Geometry: see drawing. Coordinates: mm, zero at the bounding-box minimum. Coordinates: 2 decimals unless noted, no trailing zeros. Write each loop counter-clockwise with the first axis right and the second up, starting at its lowest first coordinate (ties: lowest second). Pieces come first, ordered by that corner, then holes. Notation, with made-up numbers: M 55,-32.75 L 67,-32.75 A21 ccw 67,-14.75 Z; hole C 67,-24 d11. An arc over 180 degrees is marked long. Answer as CSV lines item,"result". Start each with the question number.
1. Section B-B on z = 3.5. Return the cut outline in (x, y).
2. Mould query, pull axis Z, two halves, no side actions, for the marked faces 1, 2, 3 and 4. Classes: pulls with the +Z half, pulls with the -Z half, needs draft (parallel to the pull), parting line crosses it, or undercut.
3. Section D-D on z = 17. Return the cut outline in (x, y).
4. Section A-A on x = 5. Return the cut outline in (y, z) (1 decimal).
5. Contact query for flat-ended pins moving along their axis: pin 1 Ø3 at (y, z) = (22, 3.5) entering from +X; pin 2 Ø2 at (x, y) = (9, 6) entering from +Z. Output: stop coordinate, or through.
6. Line query: probe 1 along Y at (x, z) = (9, 12.25); probe 2 along Y at (x, z) = (12.5, 4.25); probe 3 along X at (y, z) = (6.5, 4.5). Output: solid intervals per line, ascending. Write a range as [from, to].
7. Section C-C on y = 12.75. Return the cut outline in (x, z).
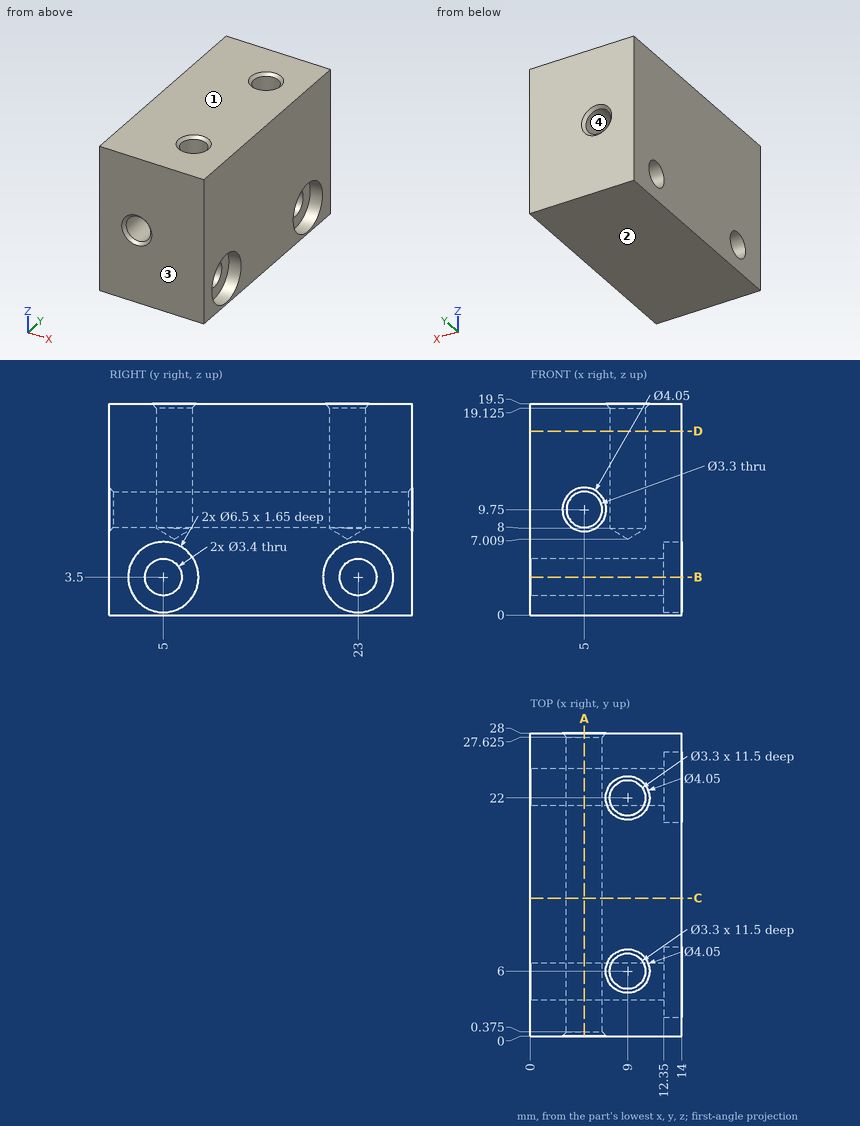
Values:
1,outline,"M 0,0 L 14,0 L 14,1.75 L 12.35,1.75 L 12.35,3.3 L 0,3.3 Z; M 0,6.7 L 12.35,6.7 L 12.35,8.25 L 14,8.25 L 14,19.75 L 12.35,19.75 L 12.35,21.3 L 0,21.3 Z; M 0,24.7 L 12.35,24.7 L 12.35,26.25 L 14,26.25 L 14,28 L 0,28 Z"
2,face 1,"pulls with the +Z half"
2,face 2,"pulls with the -Z half"
2,face 3,"needs draft"
2,face 4,"undercut"
3,outline,"M 0,0 L 14,0 L 14,28 L 0,28 Z; hole C 9,6 d3.3; hole C 9,22 d3.3"
4,outline,"M 0,0 L 28,0 L 28,7.7 L 27.6,8.1 L 0.4,8.1 L 0,7.7 Z; M 0,11.8 L 0.4,11.4 L 27.6,11.4 L 28,11.8 L 28,19.5 L 0,19.5 Z; hole C 5,3.5 d3.4; hole C 23,3.5 d3.4"
5,pin 1,"x = 12.35"
5,pin 2,"z = 7.61"
6,probe 1,"[0, 4.35], [7.65, 20.35], [23.65, 28]"
6,probe 2,"[0, 1.84], [8.16, 19.84], [26.16, 28]"
6,probe 3,"[0, 12.35]"
7,outline,"M 0,0 L 14,0 L 14,19.5 L 0,19.5 Z; hole C 5,9.75 d3.3"
